from build123d import *

# Parameters (mm, degrees)
CIRPATTERN1_COUNT = 2
CIRPATTERN1_ANGLE = 90


with BuildPart() as part:
    # Sketch1 → Revolve1 (revolve)
    with BuildSketch(Plane(origin=(0, 0, 0), x_dir=(0, 0, -1), z_dir=(1, 0, 0)), mode=Mode.PRIVATE) as revolve1_sk:
        Polygon((-51.442018331, 125.566457335), (-40.835416614, 114.959855617), (-36.769552622, 119.025719609), (-22.627416998, 104.883583986), (-24.04163056, 103.469370423), (-36.769552622, 116.197292485), (-40.835416614, 112.131428493), (-52.856231894, 124.152243773), align=None)
    revolve1 = revolve(revolve1_sk.sketch.rotate(Axis((0, 92.155661924, 0), (0, 0.7071067811865461, 0.707106781186549)), 180), axis=Axis((0, 92.155661924, 0), (0, 0.7071067811865461, 0.707106781186549)))


with BuildPart() as cirpattern1_1:
    # CirPattern1: Revolve1 ×2 about axis
    cirpattern1_axis = Axis((0, 46.077830962, -46.077830962), (0, -0.707106781, -0.707106781))
    for i in range(1, CIRPATTERN1_COUNT):
        add(revolve1.rotate(cirpattern1_axis, i * CIRPATTERN1_ANGLE / (CIRPATTERN1_COUNT - 1)))


with BuildPart() as part_1:
    add(part.part)

    # CirPattern1 united with what the copies: union CirPattern1_1
    add(cirpattern1_1.part)


solid = part_1.part
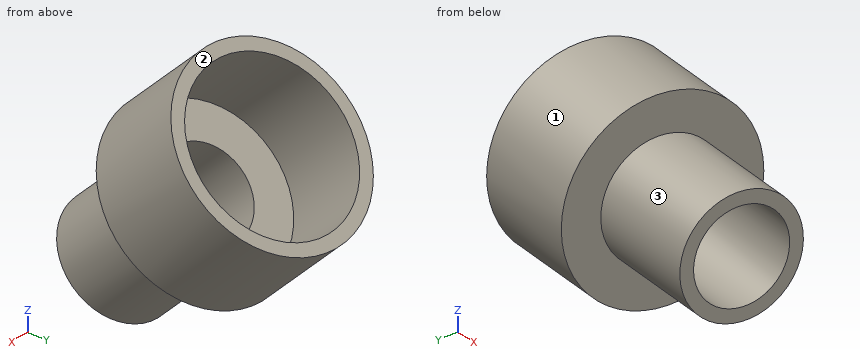
Verification items for the finished model (mm, model axes). Face numbers are marked on the shaded views. Coordinates: 2 decimals unless noted, no trailing zeros. Write each loop counter-clockwise with the first axis right and the second up, starting at its lowest first coordinate (ties: lowest second). Pieces come first, ordered by that corner, then holes. Notation, with made-up numbers: (4, 82) -> (63, 82) arc R21 cw to (63, 114) -> close; hole circle Ø11 at (-28.5, 41). An arc over 180 degrees is marked (long way). One line per item, written item: value. Start each with the question number.
Q1. Mould release check, pull along Y, two halves, no side actions. Record for the marked faces 1, 2 and 3: pulls with the +Y half, pulls with the -Y half, needs draft (parallel to the pull), parting line crosses it, or undercut.
Q2. Thickness scan on L1, parallel to Z at x = 5.5, y = 117; L2, parallel to X at y = 123, z = 30.5; L3, parallel to Z at x = -3.25, y = 114. Record the ranges inside material, lowest first. Write a range as from..to.
Q3. Go/stop test with flat-tipped pins: P1, Ø2, axis at x = -2.5, y = 140.5, coming from the -Z side; P2, Ø5, axis at y = 120.5, z = 15.5, coming from the +X side; P3, Ø12, axis at x = 4.5, z = 48.5, coming from the +Y side. Record where each tip stops, or that it passes through.
Q4. Cross-section at D-D on z = 25. State how many separate pieces and enclosed holes the cut face has, and give its area (3 significant figures).
Q5. Cross-section at A-A on x = -2. Enter the section's corners in (y, z), and give its area (3 significant figures).
Q6. Cross-section at B-B on x = -7.75. Enter the section's corners in (y, z).
Q7. Cross-section at C-C on x = 6. Enter the section's corners in (y, z).
Checked values:
1. face 1: parting line crosses it
1. face 2: pulls with the +Y half
1. face 3: undercut
2. L1: z = 14.77..18.72, 30.97..34.92, 35.97..38.8, 41.11..44.2
2. L2: x = -14.75..-7, 7..14.75
2. L3: z = 30.61..33.71, 38.97..42.19
3. P1: stops at z = 26.76
3. P2: stops at x = 6.14
3. P3: stops at y = 129.4
4. separate pieces: 1
4. enclosed holes: 2
4. area: 259 mm²
5. outline: (103.63, 23.88) -> (105.09, 22.42) -> (119.23, 36.56) -> (115.07, 40.72) -> (125.68, 51.33) -> (124.25, 52.76) -> (112.23, 40.74) -> (116.36, 36.61) -> close; (114.58, 12.93) -> (116.04, 11.47) -> (128.77, 24.2) -> (132.89, 20.07) -> (144.92, 32.09) -> (143.49, 33.52) -> (132.88, 22.92) -> (128.72, 27.08) -> close
5. area: 167 mm²
6. outline: (106.6, 20.91) -> (113.07, 14.44) -> (125.8, 27.17) -> (131.44, 21.53) -> (143.46, 33.55) -> (141.74, 35.27) -> (131.13, 24.66) -> (116.82, 38.98) -> (127.42, 49.59) -> (125.71, 51.3) -> (113.69, 39.28) -> (119.33, 33.64) -> close
7. outline: (105.09, 22.42) -> (107.28, 20.23) -> (121.43, 34.37) -> (116.02, 39.77) -> (126.63, 50.38) -> (125.05, 51.95) -> (113.03, 39.93) -> (117.82, 35.15) -> close; (112.38, 15.13) -> (114.58, 12.93) -> (127.3, 25.66) -> (132.09, 20.88) -> (144.11, 32.9) -> (142.54, 34.47) -> (131.93, 23.86) -> (126.52, 29.27) -> close
